The listing builds one solid part. Answer for the finished solid, in the listing's coordinates (mm). A direction names the side the tool comes from. Give positions to 0.01 mm unless a question says otherwise; leave off trailing zeros. Loops run counter-clockwise (first coordinate to the right, second up) from the corner with the lowest first, then second, coordinate; pieces in that order, holes last.
Item 1: The mould has two halves that part along X. Classify faces 5 (the face through (48.127, -27.815, 54.048)), 6 (the face through (25, 4, 38)), 7 (the face through (9.57, 5.97, 39.8)), 8 (the face through (46.2, -89, 61)): pulls with the +X half, pulls with the -X half, needs draft (parallel to the pull), parting line crosses it, or undercut.
Item 2: A tool of negligible diameter and unlimited length cuts with its end or side. For faces 1 (the face through (3.8, -11, 55)), 2 (the face through (25, -100, 6)), 3 (the face through (29.436, -105.465, 12.307)), 4 (the face through (25.572, 5.972, 66.787)), from which of +Z, -Z, +X, -X, +Y, -Y can it reach the whole face along a straight path? Write none if from no direction.
Item 3: Section C-C, the plane x = 44 is taken. Give the vertices of the cut face in (y, z).
Item 4: Section B-B, the plane z = 54.5 is taken. Give the vertices of the cut face in (x, y).
Item 5: Section D-D, the plane z = 38.3 is taken. Give the vertices of the cut face in (x, y), and give its area (3 significant figures).
Item 6: Section A-A, the plane x = 9.5 is taken. Give the vertices of the cut face in (y, z).
Item 7: Consider line 1 along Z through (x, y) = (16, -99); line 2 along X through (y, z) = (-26.5, 69.5); line 3 along Y through (x, z) = (25, 29.5). Determine where each line is inside the solid, lowest interval first.
Item 8: Each of these flat-tipped pins is pushed along its axis until it touches: pin 1 Ø1.5 at (x, y) = (32, -96.5) entering from -Z; pin 2 Ø3 at (x, z) = (25, 10) entering from -Y; pin 3 Ø3 at (x, y) = (32.5, -86.5) entering from -Z; pin 4 Ø12 at (y, z) = (-88, 45) entering from -X. Where does it stop, or does it pass through?
from build123d import *

# Parameters (mm, degrees)
SKETCH_1_W          = 50
SKETCH_1_H          = 20
EXTRUDE_1_DEPTH     = 8
SKETCH_2_W          = 50
SKETCH_2_H          = 4
EXTRUDE_2_DEPTH     = 13
SKETCH_3_W          = 50
SKETCH_3_H          = 60
EXTRUDE_3_DEPTH     = 4
SKETCH_4_W          = 50
SKETCH_4_H          = 5
EXTRUDE_4_DEPTH     = 40
EXTRUDE_5_DEPTH     = 50
SKETCH_7_W          = 4
SKETCH_7_H          = 5
CUT_EXTRUDE_1_DEPTH = 50
EXTRUDE_7_DEPTH     = 3.8
EXTRUDE_8_DEPTH     = 3.8
SKETCH_11_R         = 1.5
SKETCH_11_R_2       = 13
CUT_EXTRUDE_2_DEPTH = 4
SKETCH_14_W         = 4
SKETCH_14_H         = 5
EXTRUDE_9_DEPTH     = 50
CUT_EXTRUDE_3_DEPTH = 50
CUT_EXTRUDE_START   = -200
SKETCH_16_R         = 2.6
CUT_EXTRUDE_4_DEPTH = 200
SKETCH_17_R         = 5
CUT_EXTRUDE_5_DEPTH = 5
CUT_EXTRUDE_START_2 = -5
SKETCH_18_R         = 5
CUT_EXTRUDE_6_DEPTH = 5
SKETCH_19_W         = 50
SKETCH_19_H         = 4
CUT_EXTRUDE_7_DEPTH = 20
SKETCH_20_W         = 50
SKETCH_20_H         = 4
CUT_EXTRUDE_8_DEPTH = 20


with BuildPart() as part:
    # 草图1 → 凸台-拉伸1 (new body)
    with BuildSketch(Plane(origin=(0, 0, 0), x_dir=(1, 0, 0), z_dir=(0, 1, 0))):
        with Locations((25, -10)):
            Rectangle(SKETCH_1_W, SKETCH_1_H)
    extrude(amount=EXTRUDE_1_DEPTH)

    # 草图2 → 凸台-拉伸2 (add)
    with BuildSketch(Plane(origin=(0, 8, 0), x_dir=(1, 0, 0), z_dir=(0, 1, 0))):
        with Locations((25, 2)):
            Rectangle(SKETCH_2_W, SKETCH_2_H)
        with Locations((25, -22)):
            Rectangle(SKETCH_2_W, SKETCH_2_H)
    extrude(amount=-EXTRUDE_2_DEPTH)

    # 草图3 → 凸台-拉伸3 (add)
    with BuildSketch(Plane(origin=(0, 8, 0), x_dir=(1, 0, 0), z_dir=(0, 1, 0))):
        with Locations((25, -50)):
            Rectangle(SKETCH_3_W, SKETCH_3_H)
    extrude(amount=-EXTRUDE_3_DEPTH)

    # 草图4 → 凸台-拉伸4 (add)
    with BuildSketch(Plane.XZ.offset(-4)):
        with Locations((25, 77.5)):
            Rectangle(SKETCH_4_W, SKETCH_4_H)
    extrude(amount=EXTRUDE_4_DEPTH)

    # 草图6 → 凸台-拉伸5 (add)
    with BuildSketch(Plane.ZY):
        Polygon((20, -100), (-4, -100), (-4, -108), (80, -108), (80, -36), (75, -36), (75, -104), (24, -104), (24, -95), (20, -95), align=None)
    extrude(amount=-EXTRUDE_5_DEPTH)

    # 草图7 → 切除-拉伸1 (cut)
    with BuildSketch(Plane.ZY):
        with Locations((-2, -2.5)):
            Rectangle(SKETCH_7_W, SKETCH_7_H)
    extrude(amount=-CUT_EXTRUDE_1_DEPTH, mode=Mode.SUBTRACT)

    # 草图8 → 凸台-拉伸7 (add)
    with BuildSketch(Plane.ZY):
        Polygon((75, -50), (75, 4), (24, 4), (24, -5), (32.5, -5), align=None)
    extrude(amount=-EXTRUDE_7_DEPTH)

    # 草图9 → 凸台-拉伸8 (add)
    with BuildSketch(Plane(origin=(50, 0, 0), x_dir=(0, 0, -1), z_dir=(1, 0, 0))):
        Polygon((-24, -5), (-24, 4), (-75, 4), (-75, -50), (-32.5, -5), align=None)
        Polygon((-32.5, -95), (-75, -50), (-75, -104), (-24, -104), (-24, -95), align=None)
    extrude(amount=-EXTRUDE_8_DEPTH)

    # 草图11 → 切除-拉伸2 (cut)
    with BuildSketch(Plane(origin=(0, 4, 0), x_dir=(-1, 0, 0), z_dir=(0, -1, 0))):
        with Locations(Location((-40.5, -38.3, 0), (0, 0, 90))):
            Circle(SKETCH_11_R)
        with Locations(Location((-9.5, -38.3, 0), (0, 0, 90))):
            Circle(SKETCH_11_R)
        with Locations(Location((-40.5, -69.3, 0), (0, 0, 90))):
            Circle(SKETCH_11_R)
        with Locations(Location((-9.5, -69.3, 0), (0, 0, 90))):
            Circle(SKETCH_11_R)
        with Locations(Location((-25, -53.8, 0), (0, 0, 90))):
            Circle(SKETCH_11_R_2)
    extrude(amount=-CUT_EXTRUDE_2_DEPTH, mode=Mode.SUBTRACT)

    # 草图14 → 凸台-拉伸9 (add)
    with BuildSketch(Plane.ZY):
        with Locations((-2, -97.5)):
            Rectangle(SKETCH_14_W, SKETCH_14_H)
        with Locations((-2, -2.5)):
            Rectangle(SKETCH_14_W, SKETCH_14_H)
    extrude(amount=-EXTRUDE_9_DEPTH)

    # 草图15 → 切除-拉伸3 (cut)
    with BuildSketch(Plane.XZ):
        with BuildLine():
            ThreePointArc((27.6, 10), (25.491679555, 12.553086606), (22.585960604, 10.965615759))
            Line((22.585960604, 10.965615759), (27.414039396, 9.034384241))
            ThreePointArc((27.414039396, 9.034384241), (27.553086606, 9.508320445), (27.6, 10))
        make_face()
        with BuildLine():
            Line((27.414039396, 9.034384241), (22.585960604, 10.965615759))
            ThreePointArc((22.585960604, 10.965615759), (24.034384241, 7.585960604), (27.414039396, 9.034384241))
        make_face()
    extrude(amount=-CUT_EXTRUDE_3_DEPTH, mode=Mode.SUBTRACT)

    # 草图16 → 切除-拉伸4 (cut)
    with BuildSketch(Plane(origin=(0, 8, 0), x_dir=(1, 0, 0), z_dir=(0, 1, 0)).offset(CUT_EXTRUDE_START)):
        with Locations(Location((25, -10, 0), (0, 0, 90))):
            Circle(SKETCH_16_R)
    extrude(amount=CUT_EXTRUDE_4_DEPTH, mode=Mode.SUBTRACT)

    # 草图17 → 切除-拉伸5 (cut)
    with BuildSketch(Plane(origin=(0, 8, 0), x_dir=(1, 0, 0), z_dir=(0, 1, 0))):
        with Locations(Location((25, -10, 0), (0, 0, 270))):
            Circle(SKETCH_17_R)
    extrude(amount=-CUT_EXTRUDE_5_DEPTH, mode=Mode.SUBTRACT)

    # 草图18 → 切除-拉伸6 (cut)
    with BuildSketch(Plane.XZ.offset(108).offset(CUT_EXTRUDE_START_2)):
        with Locations(Location((25, 10, 0), (0, 0, 90))):
            Circle(SKETCH_18_R)
    extrude(amount=CUT_EXTRUDE_6_DEPTH, mode=Mode.SUBTRACT)

    # 草图19 → 切除-拉伸7 (cut)
    with BuildSketch(Plane(origin=(0, -5, 0), x_dir=(-1, 0, 0), z_dir=(0, -1, 0))):
        with Locations((-25, 2)):
            Rectangle(SKETCH_19_W, SKETCH_19_H)
    extrude(amount=-CUT_EXTRUDE_7_DEPTH, mode=Mode.SUBTRACT)

    # 草图20 → 切除-拉伸8 (cut)
    with BuildSketch(Plane(origin=(0, -95, 0), x_dir=(1, 0, 0), z_dir=(0, 1, 0))):
        with Locations((25, 2)):
            Rectangle(SKETCH_20_W, SKETCH_20_H)
    extrude(amount=-CUT_EXTRUDE_8_DEPTH, mode=Mode.SUBTRACT)


solid = part.part
Worked answers:
1. face 5: needs draft
1. face 6: undercut
1. face 7: undercut
1. face 8: pulls with the -X half
2. face 1: none
2. face 2: -Z, +X, -X
2. face 3: -Y
2. face 4: +Y
3. outline: (-108, 0) - (-100, 0) - (-100, 20) - (-95, 20) - (-95, 24) - (-104, 24) - (-104, 75) - (4, 75) - (4, 24) - (-5, 24) - (-5, 20) - (0, 20) - (0, 0) - (8, 0) - (8, 80) - (-108, 80) - close
4. outline: (0, -108) - (50, -108) - (50, -71.71) - (46.2, -71.71) - (46.2, -104) - (0, -104) - close; (0, -28.29) - (3.8, -28.29) - (3.8, 4) - (12.02, 4) - (12.02, 8) - (0, 8) - close; (37.98, 4) - (46.2, 4) - (46.2, -28.29) - (50, -28.29) - (50, 8) - (37.98, 8) - close
5. outline: (0, -108) - (50, -108) - (50, -88.86) - (46.2, -88.86) - (46.2, -104) - (0, -104) - close; (0, -11.14) - (3.8, -11.14) - (3.8, 4) - (8, 4) - (8, 8) - (0, 8) - close; (11, 4) - (39, 4) - (39, 8) - (11, 8) - close; (42, 4) - (46.2, 4) - (46.2, -11.14) - (50, -11.14) - (50, 8) - (42, 8) - close
5. area: 549 mm2
6. outline: (-108, 0) - (-100, 0) - (-100, 20) - (-95, 20) - (-95, 24) - (-104, 24) - (-104, 75) - (4, 75) - (4, 70.8) - (8, 70.8) - (8, 80) - (-108, 80) - close; (-5, 20) - (0, 20) - (0, 0) - (8, 0) - (8, 36.8) - (4, 36.8) - (4, 24) - (-5, 24) - close; (4, 39.8) - (8, 39.8) - (8, 67.8) - (4, 67.8) - close
7. line 1: z = 20 to 24, 75 to 80
7. line 2: x = 0 to 3.8, 46.2 to 50
7. line 3: y = -108 to -104, 4 to 8
8. pin 1: stops at z = 20
8. pin 2: passes through
8. pin 3: stops at z = 75
8. pin 4: stops at x = 46.2
